Work out the finished part from the listing and answer in its coordinate system (mm). A direction names the side the tool comes from. Coordinates: 2 decimals unless noted, no trailing zeros. Order: outer loops, then holes, each group sorted by start corner. A loop starts at its lowest first (then second) coordinate and runs counter-clockwise, first axis right, second up. Notation, with made-up numbers: (33.25, 60) -> (72.25, 60) arc R14 cw to (72.25, 74) -> close; hole circle Ø9 at (54, 14). An arc over 180 degrees is marked (long way). Answer as CSV lines item,"result". Start each with the question number.
Item 1: Which of the six approach directions +Z, -Z, +X, -X, +Y, -Y give full straight-line access (tool end or side, diameter ignored) to faces 1 (the face through (10.1, 0, 7.6)), 2 (the face through (10, 63, 13.9)), 3 (the face through (15.209, 62.611, 5.846))?
Item 2: Straight lines are drawn through the part: L1, parallel to Z at x = 1.75, y = 30 (3 decimals); L2, parallel to X at y = 84.5, z = 10; L3, parallel to Z at x = 14.25, y = 33.5 (3 decimals). For each, find the intervals that lie inside material, in ascending order.
Item 3: Each of these flat-tipped pins is pushed along its axis until it touches: pin 1 Ø6 at (y, z) = (43, 10) entering from +X; pin 2 Ø6.5 at (x, y) = (9.5, 74) entering from +Z; pin 3 Ø4.5 at (y, z) = (49, 9.5) entering from -X. Where does it stop, or does it pass through?
Item 4: For a pull along Z with two mould halves and no side action, classify faces 4 (the face through (5.843, 62.611, 4.788)), 5 (the face through (10.1, 127, 7.6)), 6 (the face through (6.1, 63, 10)), 7 (the face through (3, 63, 0)) as pulls with the +Z half, pulls with the -Z half, needs draft (parallel to the pull), parting line crosses it, or undercut.
Item 5: Section B-B (z = 10) is taken. Write down the section's boundary in (x, y).
Item 6: Section A-A (x = 10) is taken. Write down the section's boundary in (y, z), then the cut area to 3 significant figures.
```python
from build123d import *

# Parameters (mm, degrees)
SKETCH2_R              = 2.074585303
VSLOT2020_2020_5_DEPTH = 127


with BuildPart() as part:
    # Sketch2 → Vslot2020 2020(5) (new body)
    with BuildSketch(Plane.ZX):
        with BuildLine():
            Line((13.9, 7.149086807), (13.9, 12.844511469))
            Line((13.9, 12.844511469), (16.558493656, 15.492177728))
            Line((16.558493656, 15.492177728), (16.550703242, 15.5))
            Line((16.550703242, 15.5), (18.2, 15.5))
            Line((18.2, 15.5), (18.2, 13.12))
            Line((18.2, 13.12), (18.534428266, 13.12))
            Line((18.534428266, 13.12), (20, 14.58))
            Line((20, 14.58), (20, 19.5))
            ThreePointArc((20, 19.5), (19.853553391, 19.853553391), (19.5, 20))
            Line((19.5, 20), (14.575, 20))
            Line((14.575, 20), (13.12, 18.545))
            Line((13.12, 18.545), (13.12, 18.2))
            Line((13.12, 18.2), (15.5, 18.2))
            Line((15.5, 18.2), (15.5, 16.555))
            Line((15.5, 16.555), (12.834142613, 13.9))
            Line((12.834142613, 13.9), (7.155, 13.9))
            Line((7.155, 13.9), (4.5, 16.555))
            Line((4.5, 16.555), (4.5, 18.2))
            Line((4.5, 18.2), (6.875, 18.2))
            Line((6.875, 18.2), (6.875, 18.545))
            Line((6.875, 18.545), (5.42, 20))
            Line((5.42, 20), (0.5, 20))
            ThreePointArc((0.5, 20), (0.146446609, 19.853553391), (0, 19.5))
            Line((0, 19.5), (0, 14.58))
            Line((0, 14.58), (1.46, 13.12))
            Line((1.46, 13.12), (1.8, 13.12))
            Line((1.8, 13.12), (1.8, 15.5))
            Line((1.8, 15.5), (3.445, 15.5))
            Line((3.445, 15.5), (3.439339828, 15.494339828))
            Line((3.439339828, 15.494339828), (6.094339828, 12.839339828))
            Line((6.094339828, 12.839339828), (6.1, 12.845))
            Line((6.1, 12.845), (6.1, 7.149086807))
            Line((6.1, 7.149086807), (3.439339828, 4.5))
            Line((3.439339828, 4.5), (1.8, 4.5))
            Line((1.8, 4.5), (1.8, 6.88))
            Line((1.8, 6.88), (1.46, 6.88))
            Line((1.46, 6.88), (0, 5.42))
            Line((0, 5.42), (0, 0.5))
            ThreePointArc((0, 0.5), (0.146446609, 0.146446609), (0.5, 0))
            Line((0.5, 0), (5.42, 0))
            Line((5.42, 0), (6.875, 1.455))
            Line((6.875, 1.455), (6.875, 1.8))
            Line((6.875, 1.8), (4.5, 1.8))
            Line((4.5, 1.8), (4.5, 3.4393348))
            Line((4.5, 3.4393348), (7.158345795, 6.086117297))
            Line((7.158345795, 6.086117297), (7.144523479, 6.1))
            Line((7.144523479, 6.1), (12.854625295, 6.1))
            Line((12.854625295, 6.1), (12.841221344, 6.086548451))
            Line((12.841221344, 6.086548451), (15.499715, 3.437461644))
            Line((15.499715, 3.437461644), (15.5, 1.8))
            Line((15.5, 1.8), (13.12, 1.8))
            Line((13.12, 1.8), (13.12, 1.455))
            Line((13.12, 1.455), (14.575, 0))
            Line((14.575, 0), (19.5, 0))
            ThreePointArc((19.5, 0), (19.853553391, 0.146446609), (20, 0.5))
            Line((20, 0.5), (20, 5.42))
            Line((20, 5.42), (18.606904708, 6.88))
            Line((18.606904708, 6.88), (18.2, 6.88))
            Line((18.2, 6.88), (18.2, 4.5))
            Line((18.2, 4.5), (16.558493656, 4.5))
            Line((16.558493656, 4.5), (13.9, 7.149086807))
        make_face()
        with Locations((10, 10)):
            Circle(SKETCH2_R, mode=Mode.SUBTRACT)
    extrude(amount=VSLOT2020_2020_5_DEPTH)


solid = part.part
```
Checked values:
1,face 1,"+Z, -Z, +X, -X, -Y"
1,face 2,"+Z, +Y, -Y"
1,face 3,"+Y, -Y"
2,L1,"z = 0 to 6.875, 13.12 to 20"
2,L2,"x = 6.1 to 7.93, 12.07 to 13.9"
2,L3,"z = 0.33 to 1.8, 4.684 to 6.805, 13.186 to 15.311, 18.2 to 19.669"
3,pin 1,"stops at x = 14.07"
3,pin 2,"stops at z = 19.21"
3,pin 3,"stops at x = 6.1"
4,face 4,"undercut"
4,face 5,"needs draft"
4,face 6,"undercut"
4,face 7,"pulls with the -Z half"
5,outline,"(6.1, 0) -> (7.93, 0) -> (7.93, 127) -> (6.1, 127) -> close; (12.07, 0) -> (13.9, 0) -> (13.9, 127) -> (12.07, 127) -> close"
6,outline,"(0, 6.1) -> (127, 6.1) -> (127, 7.93) -> (0, 7.93) -> close; (0, 12.07) -> (127, 12.07) -> (127, 13.9) -> (0, 13.9) -> close"
6,area,"464 mm^2"
